Input: part model. Units: mm. Frame: model coordinates. A direction names the side the tool comes from. Give positions to 0.01 mm unless a question says otherwise; leave off trailing zeros. Order: outer loops, then holes, each group sorted by start corner. A loop starts at its lowest first (then second) coordinate and runs counter-clockwise, first axis right, second up. Notation, with made-up numbers: M 49,-19.75 L 62,-19.75 A31 cw 62,4.25 Z; hole C 11,-26.75 d6. An arc over 180 degrees is marked long. Use a Markdown table: item, result.
from build123d import *

# Parameters (mm, degrees)
EXTRUDE1_DEPTH = 7
EXTRUDE2_DEPTH = 20.3


with BuildPart() as part:
    # Sketch1 → Revolve1 (revolve)
    with BuildSketch(Plane.XY, mode=Mode.PRIVATE) as revolve1_sk:
        with BuildLine():
            Line((6, 31.680378901), (8.05, 31.680378901))
            Line((8.05, 31.680378901), (8.05, 19.880378901))
            ThreePointArc((8.05, 19.880378901), (8.55, 19.380378901), (8.05, 18.880378901))
            Line((8.05, 18.880378901), (8.05, 17.080378901))
            Line((8.05, 17.080378901), (3.5, 17.080378901))
            Line((3.5, 17.080378901), (3.5, 15.680378901))
            Line((3.5, 15.680378901), (2.5, 15.680378901))
            Line((2.5, 15.680378901), (2.5, 2.980378901))
            Line((2.5, 2.980378901), (0, 2.980378901))
            Line((0, 2.980378901), (0, 20.880378901))
            Line((0, 20.880378901), (0.5, 20.880378901))
            add(Edge.make_bspline(
                [(0.5, 20.880378901), (0.932106432, 20.906651763), (1.887530423, 20.96474329), (3.549630763, 21.874391527), (4.219232089, 24.338558209), (4.618386004, 26.623285295), (4.718036301, 28.180794336), (4.75, 28.680378901)],
                knots=[0, 0, 0, 0, 0.130075309, 0.287607547, 0.531387804, 0.849688564, 1, 1, 1, 1], degree=3))
            Line((4.75, 28.680378901), (6, 31.580378901))
            Line((6, 31.580378901), (6, 31.680378901))
        make_face()
    revolve(revolve1_sk.sketch.rotate(Axis((0, 0, 0), (0, 1, 0)), 90), axis=Axis((0, 0, 0), (0, 1, 0)))  # turned: the seam where the file's is

    # Sketch2 → Extrude1 (cut)
    with BuildSketch(Plane.XZ.offset(-2.980378901)):
        Polygon((1.785357107, 1.75), (4.264804166, 1.75), (0.483637586, 4.675163329), (-4.469983747, 1.75), align=None)
        Polygon((-4.469983747, -1.75), (4.264804166, -1.75), (0.383778189, -4.04178496), align=None)
    extrude(amount=-EXTRUDE1_DEPTH, mode=Mode.SUBTRACT)

    # Sketch3 → Extrude2 (cut, through all)
    with BuildSketch(Plane.XY.offset(10.75)):
        with BuildLine():
            Line((-1.55, 37.698212451), (1.55, 37.698212451))
            Line((1.55, 37.698212451), (1.55, 24.130378901))
            ThreePointArc((1.55, 24.130378901), (0, 22.580378901), (-1.55, 24.130378901))
            Line((-1.55, 24.130378901), (-1.55, 37.698212451))
        make_face()
    extrude(amount=-EXTRUDE2_DEPTH, mode=Mode.SUBTRACT)


solid = part.part
1) First-contact query: pin 1 Ø3 at (x, y) = (-2, 15) entering from -Z; pin 2 Ø8 at (x, y) = (-6, 16.5) entering from -Z; pin 3 Ø3.5 at (y, z) = (28.5, 6.5) entering from -X. Flat tips, straight axial feed; report the tip coordinate or a pass-through.
Response values:
| item | result |
|---|---|
| pin 1 | stops at z = -3.44 |
| pin 2 | stops at z = -7.95 |
| pin 3 | stops at x = -6.5 |
2) Material intervals for line 1 (Y direction, x = -4.75, z = 4.75); line 2 (X direction, y = 30.75, z = 4.25); line 3 (Y direction, x = -0.25, z = -0.5), sorted ascending. Write a range as from..to.
Response values:
| item | result |
|---|---|
| line 1 | y = 17.08..31.68 |
| line 2 | x = -6.84..-3.71, 3.71..6.84 |
| line 3 | y = 2.98..20.88 |
3) Cut plane A-A on y = 10.75. Return loops of the section in (x, z).
Response values:
| item | result |
|---|---|
| outline | C 0,0 d5 |
4) Mould query, pull axis Z, two halves, no side actions, for faces 1 (the face through (0, 20.88, 0)), 2 (the face through (-1.55, 28, -6)), 3 (the face through (0, 6, 1.75)). Classes: released by +Z, released by -Z, zero draft, split by the parting line, or undercut.
Response values:
| item | result |
|---|---|
| face 1 | undercut |
| face 2 | zero draft |
| face 3 | released by +Z |
5) Reachability of faces 4 (the face through (1.55, 28, -6)), 5 (the face through (5.105, 29.506, 0.094)), 6 (the face through (-2.418, 17.968, -7.678)) from +Z, -Z, +X, -X, +Y, -Y: full face, straight path, thin tool, end or side. Return the list, or none.
Response values:
| item | result |
|---|---|
| face 4 | +Z, -Z, +Y |
| face 5 | +Y |
| face 6 | -Y |
